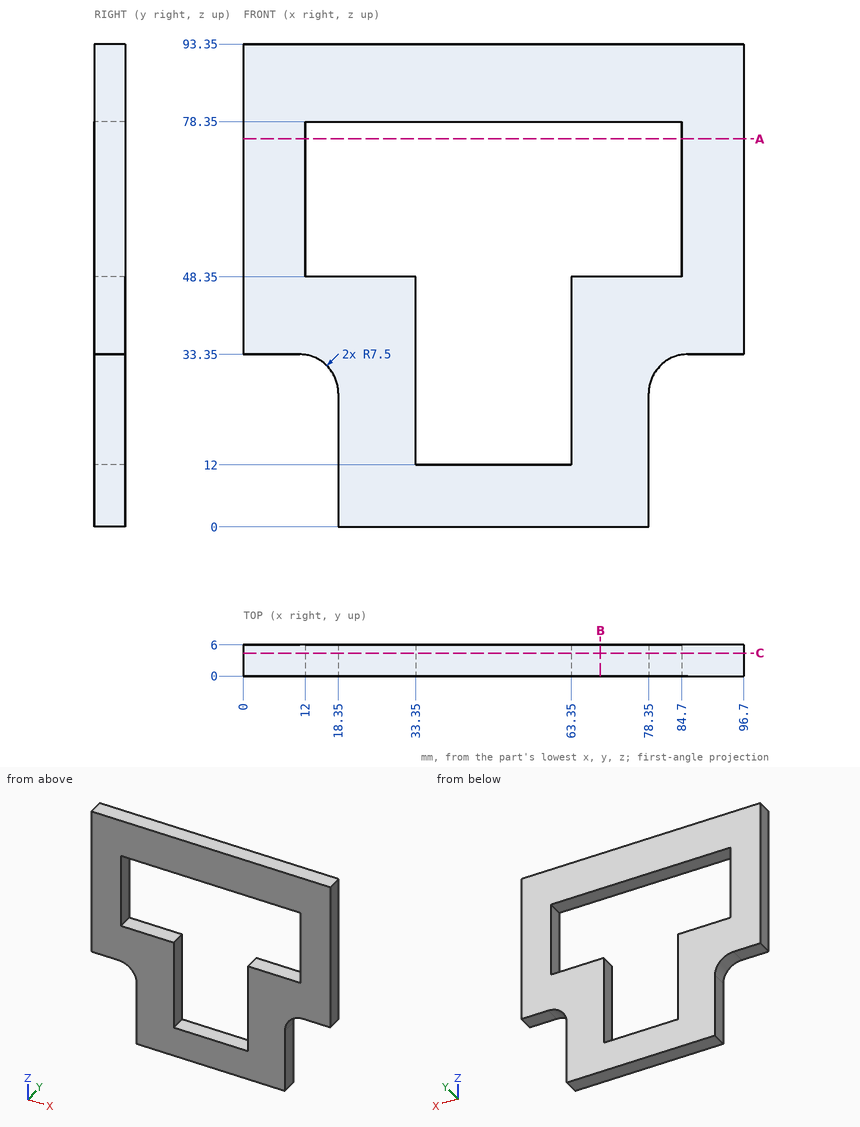
Answer from the drawing. Dimensions are ordinates in mm from the lowest x, y and z of the part. Coordinates: 2 decimals unless noted, no trailing zeros. Loops run counter-clockwise (first coordinate to the right, second up) from the corner with the lowest first, then second, coordinate; pieces in that order, holes last. Notation, with made-up numbers: (-37, -28.5) -> (17, -28.5) arc R24 ccw to (17, -4.5) -> close; hole circle Ø4 at (61.25, 59.25). An arc over 180 degrees is marked (long way). Return JSON: item names as keys, results as strings.
Item 1: Flat-ended cylindrical pins translate along their axes: P1, Ø3, axis at x = 89.5, y = 3.5, coming from the -Z side; P2, Ø1.8, axis at y = 1.5, z = 30, coming from the +X side; P3, Ø1, axis at x = 85, y = 1, coming from the -Z side; P4, Ø3, axis at x = 44.5, z = 15, coming from the +Y side. Find the tip coordinate at first contact, or state that the pin passes through.
Answers:
{"P1": "stops at z = 33.35", "P2": "stops at x = 80.3", "P3": "stops at z = 33.23", "P4": "passes through"}
Item 2: Find the intervals of material crossed by probe 1 along X at (y, z) = (3.85, 21.5); probe 2 along X at (y, z) = (3.25, 40); probe 3 along Z at (x, y) = (67.5, 4.45), in increasing order.
Answers:
{"probe 1": "x = 18.35 to 33.35, 63.35 to 78.35", "probe 2": "x = 0 to 33.35, 63.35 to 96.7", "probe 3": "z = 0 to 48.35, 78.35 to 93.35"}
Item 3: Find section B-B (x = 69). Determine the outline of the cut face in (y, z), plus the area to 3 significant figures.
Answers:
{"outline": "(0, 0) -> (6, 0) -> (6, 48.35) -> (0, 48.35) -> close; (0, 78.35) -> (6, 78.35) -> (6, 93.35) -> (0, 93.35) -> close", "area": "380 mm2"}
Item 4: Find section A-A (z = 75). Determine the outline of the cut face in (x, y).
Answers:
{"outline": "(0, 0) -> (12, 0) -> (12, 6) -> (0, 6) -> close; (84.7, 0) -> (96.7, 0) -> (96.7, 6) -> (84.7, 6) -> close"}
Item 5: Find section C-C (y = 4.4). Determine the outline of the cut face in (x, z).
Answers:
{"outline": "(0, 33.35) -> (10.85, 33.35) arc R7.5 cw to (18.35, 25.85) -> (18.35, 0) -> (78.35, 0) -> (78.35, 25.85) arc R7.5 cw to (85.85, 33.35) -> (96.7, 33.35) -> (96.7, 93.35) -> (0, 93.35) -> close; hole (12, 48.35) -> (33.35, 48.35) -> (33.35, 12) -> (63.35, 12) -> (63.35, 48.35) -> (84.7, 48.35) -> (84.7, 78.35) -> (12, 78.35) -> close"}
